Geometry check sheet. Reference: drawing and pictorial views, mm from the part's lowest x, y, z. A direction names the side the tool comes from. Round coordinates to 2 decimals unless told otherwise and drop trailing zeros. Write each loop counter-clockwise with the first axis right and the second up, starting at its lowest first coordinate (ties: lowest second). Pieces come first, ordered by that corner, then holes. Notation, with made-up numbers: M -20.5,71.25 L 9.5,71.25 A21 ccw 9.5,95.25 Z; hole C -2,60 d6. An arc over 180 degrees is marked long. Answer in a Markdown table with one row per item.
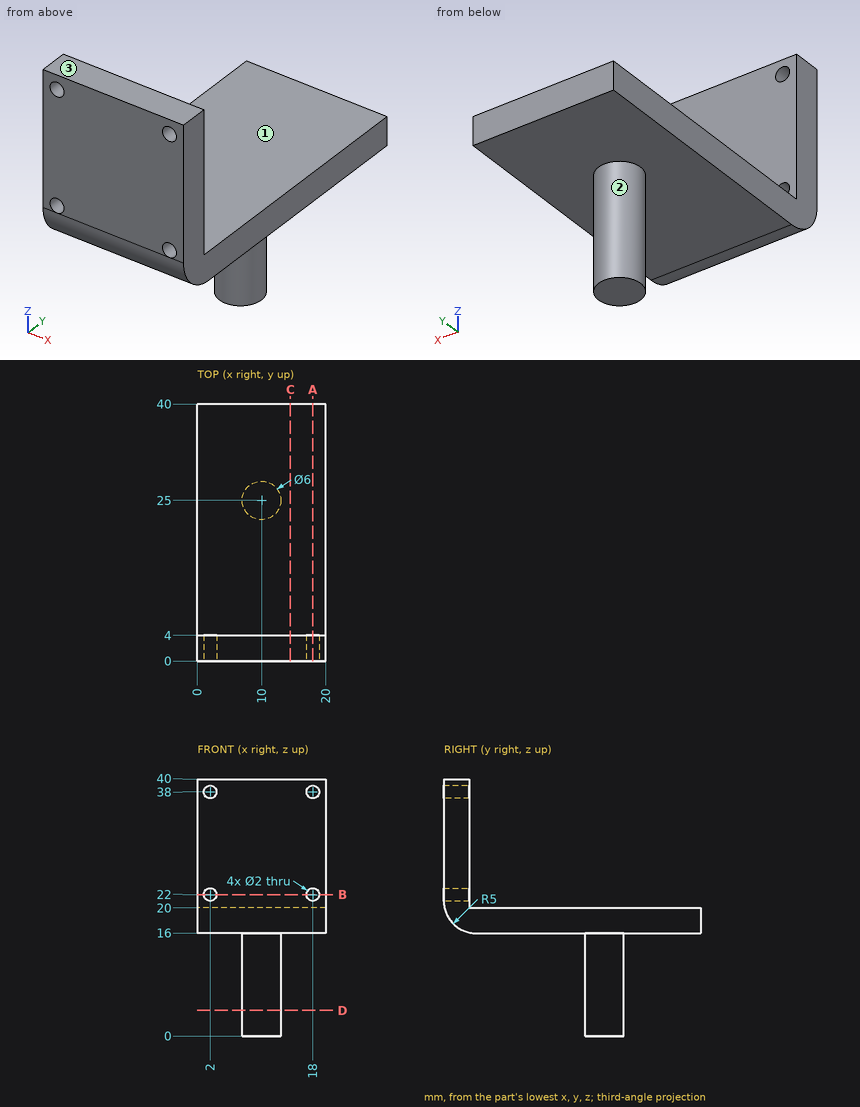
1. Section check A-A, the plane x = 18. Count the separate pieces of the cut face and the enclosed holes in it, and give its area (3 significant figures).
Found:
| item | result |
|---|---|
| separate pieces | 3 |
| enclosed holes | 0 |
| area | 219 mm2 |
2. Section check C-C, the plane x = 14.5. Record the cut outline in (y, z).
Found:
| item | result |
|---|---|
| outline | M 0,21 A5 ccw 5,16 L 40,16 L 40,20 L 4,20 L 4,40 L 0,40 Z |
3. Section check D-D, the plane z = 4. Record the cut outline in (x, y), and give its area (3 significant figures).
Found:
| item | result |
|---|---|
| outline | C 10,25 d6 |
| area | 28.3 mm2 |
4. Scan lines: L1, parallel to X at y = 1.4, z = 22; L2, parallel to Z at x = 2.25, y = 3.5; L3, parallel to Z at x = 7.5, y = 32.5. Record each from-to range of solid material in increasing order.
Found:
| item | result |
|---|---|
| L1 | x = 0 to 1, 3 to 17, 19 to 20 |
| L2 | z = 16.23 to 21.03, 22.97 to 37.03, 38.97 to 40 |
| L3 | z = 16 to 20 |
5. Go/stop test with flat-tipped pins: pin 1 (2.5 mm diameter, centred on x = 2, z = 38, fed in from +Y); pin 2 (10 mm diameter, centred on x = 7.5, y = 35.5, fed in from -Z); pin 3 (8 mm diameter, centred on x = 11, y = 23.5, fed in from -Z); pin 4 (1 mm diameter, centred on x = 3, y = 9.5, fed in from +Z). Record where each tip stops, or that it passes through.
Found:
| item | result |
|---|---|
| pin 1 | stops at y = 4 |
| pin 2 | stops at z = 16 |
| pin 3 | stops at z = 0 |
| pin 4 | stops at z = 20 |
6. Section check B-B, the plane z = 22. Record the cut outline in (x, y), and give its area (3 significant figures).
Found:
| item | result |
|---|---|
| outline | M 0,0 L 1,0 L 1,4 L 0,4 Z; M 3,0 L 17,0 L 17,4 L 3,4 Z; M 19,0 L 20,0 L 20,4 L 19,4 Z |
| area | 64.0 mm2 |
7. Access from +Z, -Z, +X, -X, +Y, -Y to the whole of each face (thin tool, end or side, straight path). Record for the marked faces 1, 2 and 3.
Found:
| item | result |
|---|---|
| face 1 | +Z, +X, -X, +Y |
| face 2 | -Z |
| face 3 | +Z, +X, -X, +Y, -Y |
